CAD build for the part. Positions are in the model's coordinates, mm. A direction names the side the tool comes from. Give positions to 0.01 mm unless a question says otherwise; leave off trailing zeros. Write each loop counter-clockwise with the first axis right and the second up, starting at its lowest first coordinate (ties: lowest second). Pieces come first, ordered by that corner, then holes. Notation, with made-up numbers: (37.25, 26.25) - (74.25, 26.25) arc R26 cw to (74.25, 48.25) - close; hole circle Ø7 at (58.5, 20). An arc over 180 degrees is marked (long way). Answer as a JSON object with one key per item and string values.
Autodesk Inventor part; units mm, degrees
ref_plane "YZ Plane" through (0, 0, 0) normal (1, 0, 0) x (0, 1, 0)
ref_plane "XZ Plane" through (0, 0, 0) normal (0, 1, 0) x (-1, 0, 0)
ref_plane "XY Plane" through (0, 0, 0) normal (0, 0, 1) x (1, 0, 0)
sketch "Sketch1" plane through (0, 0, 0) normal (0, 0, 1) x (1, 0, 0)
  line L0 (23.0237, 36.3892) -> (128.0237, 36.3892)
  line L1 (128.0237, 36.3892) -> (128.0237, 16.3892)
  line L2 (128.0237, 16.3892) -> (23.0237, 16.3892)
  line L3 (23.0237, 16.3892) -> (23.0237, 36.3892)
  line L4 (33.0237, 16.3892) -> (53.0237, 16.3892)
  line L5 (53.0237, 16.3892) -> (53.0237, 11.3892)
  line L6 (53.0237, 11.3892) -> (33.0237, 11.3892)
  line L7 (33.0237, 11.3892) -> (33.0237, 16.3892)
  line L8 (98.0237, 16.3892) -> (118.0237, 16.3892)
  line L9 (118.0237, 16.3892) -> (118.0237, 11.3892)
  line L10 (118.0237, 11.3892) -> (98.0237, 11.3892)
  line L11 (98.0237, 11.3892) -> (98.0237, 16.3892)
  point P0 (0, 0)
  point P1 (33.0237, 13.8892)
  dimension "d0" = 105
  dimension "d1" = 20
  dimension "d2" = 20
  dimension "d3" = 5
  dimension "d4" = 20
  dimension "d5" = 5
  dimension "d6" = 10
  dimension "d7" = 10
extrude "Extrusion1" add sketch "Sketch1" along normal blind 5
properties part number "inslide2"
(1) Pull direction X, two halves, no side cores. Call faces 6 (the face through (118.024, 14, 2)), 7 (the face through (75, 36.389, 2)), 8 (the face through (98.024, 14, 2)): pulls with the +X half, pulls with the -X half, needs draft (parallel to the pull), parting line crosses it, or undercut.
Answer key:
{"face 6": "pulls with the +X half", "face 7": "needs draft", "face 8": "undercut"}
(2) Probe L1, parallel to X at y = 14.25, z = 3.55; L2, parallel to Y at x = 86, z = 2.1. List the from-to ranges inside material, lowest first. Write a range as [from, to].
Answer key:
{"L1": "x = [33.02, 53.02], [98.02, 118.02]", "L2": "y = [16.39, 36.39]"}
(3) 3-axis set-ups, long thin cutter, end or side, ignore diameter. For faces 1 (the face through (123, 16.389, 2)), 2 (the face through (53.024, 14, 2)), 3 (the face through (75, 24, 5)), 4 (the face through (28, 16.389, 2)), 5 (the face through (43, 11.389, 2)): which of +Z, -Z, +X, -X, +Y, -Y reach the whole face in a straight line?
Answer key:
{"face 1": "+Z, -Z, +X, -Y", "face 2": "+Z, -Z, -Y", "face 3": "+Z, +X, -X, +Y, -Y", "face 4": "+Z, -Z, -X, -Y", "face 5": "+Z, -Z, +X, -X, -Y"}
(4) Saw through at C-C, the plane x = 71.5. Give the cut face in (y, z), and give its area (3 significant figures).
Answer key:
{"outline": "(16.39, 0) - (36.39, 0) - (36.39, 5) - (16.39, 5) - close", "area": "100 mm²"}
(5) Saw through at A-A, the plane y = 13.5. Give the cut face in (x, z), and give its area (3 significant figures).
Answer key:
{"outline": "(33.02, 0) - (53.02, 0) - (53.02, 5) - (33.02, 5) - close; (98.02, 0) - (118.02, 0) - (118.02, 5) - (98.02, 5) - close", "area": "200 mm²"}
(6) Flat gauge pin, fed straight in: P1, Ø1.5, axis at x = 26, z = 3, coming from the -Y side. Where does the tip first touch, or does it go through?
Answer key:
{"P1": "stops at y = 16.39"}
(7) Saw through at B-B, the plane z = 1.7. Give the cut face in (x, y), and give its area (3 significant figures).
Answer key:
{"outline": "(23.02, 16.39) - (33.02, 16.39) - (33.02, 11.39) - (53.02, 11.39) - (53.02, 16.39) - (98.02, 16.39) - (98.02, 11.39) - (118.02, 11.39) - (118.02, 16.39) - (128.02, 16.39) - (128.02, 36.39) - (23.02, 36.39) - close", "area": "2,300 mm²"}
